Input: part model. Units: mm. Frame: model coordinates. Face numbers are marked on the shaded views. A direction names the side the tool comes from. Round coordinates to 2 decimals unless told otherwise and drop trailing zeros. Loops run counter-clockwise (first coordinate to the right, second up) from the corner with the lowest first, then second, coordinate; pieces in that order, holes last. Notation, with made-up numbers: (-25.75, 84.25) - (-15.75, 84.25) arc R13 ccw to (-15.75, 104.25) - close; hole circle Ø4 at (68, 45.5). An arc over 180 degrees is marked (long way). Write each question's results on one line, items separated by ' | '.
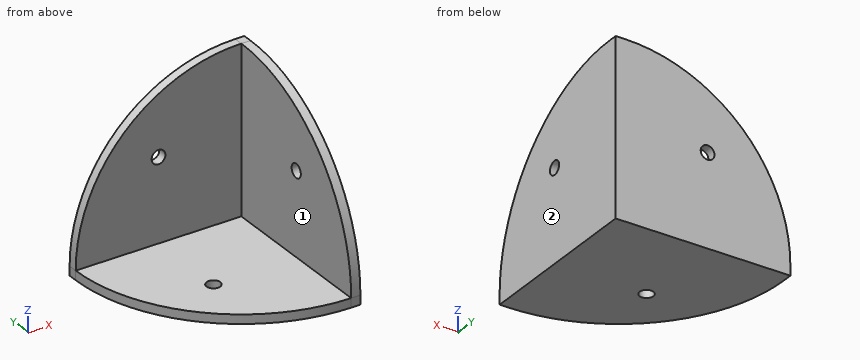
Autodesk Fusion 360 part; units mm, degrees
sketch "Sketch3" plane through (0, 0, 0) normal (0, 0, 1) x (1, 0, 0)
  line L0 (10, 15) -> (46, 15)
  line L1 (46, 15) -> (46, 51)
  line L2 (46, 51) -> (10, 51)
  line L3 (10, 51) -> (10, 15)
  line L4 (8, 53) -> (8, 13)
  line L5 (8, 13) -> (48, 13)
  line L6 (48, 13) -> (48, 53)
  line L7 (48, 53) -> (8, 53)
  line L8 (10, 51) -> (10, 53)
  line L9 (10, 51) -> (8, 51)
  line L10 (46, 51) -> (46, 53)
  line L11 (46, 51) -> (48, 51)
  line L12 (46, 15) -> (48, 15)
  line L13 (46, 15) -> (46, 13)
  line L14 (10, 15) -> (10, 13)
  line L15 (10, 15) -> (8, 15)
  dimension "d6" = 36
  dimension "d7" = 36
  dimension "d8" = 2
extrude "Extrude1" add sketch "Sketch3" along normal blind 38 contours L1 L6 L11 L12 | L2 L7 L8 L10 | L6 L7 L10 L11
extrude "Extrude2" add sketch "Sketch3" along normal blind 2 contours L0 L1 L2 L3
sketch "Sketch4" plane through (0, 0, 2) normal (0, 0, 1) x (-1, 0, 0)
  line L0 (-10, -51) -> (-10, -15)
  line L1 (-10, -15) -> (-46, -15)
  line L2 (-46, -15) -> (-46, -51)
  line L3 (-46, -51) -> (-10, -51)
  line L4 (-10, -51) -> (-46, -15)
  line L5 (-10, -15) -> (-46, -51)
  circle A0 centre (-28, -33) radius 1.5
  dimension "d13" = 3
sketch "Sketch5" plane through (0, 51, 0) normal (0, -1, 0) x (1, 0, 0)
  line L0 (10, 2) -> (46, 2)
  line L1 (46, 2) -> (46, 38)
  line L2 (46, 38) -> (10, 38)
  line L3 (10, 38) -> (10, 2)
  line L4 (10, 38) -> (46, 2)
  line L5 (10, 2) -> (46, 38)
  circle A0 centre (28, 20) radius 1.5
  dimension "d14" = 3
sketch "Sketch6" plane through (46, 0, 0) normal (-1, 0, 0) x (0, -1, 0)
  line L0 (-51, 2) -> (-15, 2)
  line L1 (-15, 2) -> (-15, 38)
  line L2 (-15, 38) -> (-51, 38)
  line L3 (-51, 38) -> (-51, 2)
  line L4 (-51, 38) -> (-15, 2)
  line L5 (-51, 2) -> (-15, 38)
  circle A0 centre (-33, 20) radius 1.5
  dimension "d15" = 3
extrude "Extrude3" cut sketch "Sketch5" against normal blind 7 contours L4 L5 A0 | L4 L5 A0 | L4 L5 A0 | L4 L5 A0
extrude "Extrude4" cut sketch "Sketch6" against normal blind 10 contours L4 L5 A0 | L4 L5 A0 | L4 L5 A0 | L4 L5 A0
extrude "Extrude5" cut sketch "Sketch4" against normal blind 9 contours L4 L5 A0 | L4 L5 A0 | L4 L5 A0 | L4 L5 A0
fillet "Fillet1" radius 36 3 edges at (10, 52, 38) (10, 15, 1) (47, 15, 38)
1. Line query: line 1 (Z direction, x = 18.5, y = 33.5); line 2 (Y direction, x = 28, z = 0.9); line 3 (Y direction, x = 44.5, z = 24). Output: solid intervals per line, ascending. Write a range as [from, to].
Answer:
line 1: [0, 2] | line 2: [19.82, 31.5], [34.5, 53] | line 3: [51, 53]
2. Section query A-A, the plane x = 28. Output: boundary loops of the cut face in (y, z).
Answer:
outline: (19.82, 0) - (31.5, 0) - (31.5, 2) - (19.82, 2) - close; (34.5, 0) - (53, 0) - (53, 18.5) - (51, 18.5) - (51, 2) - (34.5, 2) - close; (51, 21.5) - (53, 21.5) - (53, 33.18) - (51, 33.18) - close
3. Set-up query: the marked faces 1 and 2. Return all of +Z, -Z, +X, -X, +Y, -Y with unobstructed straight access to the full face (end or side cutting, diameter ignored); none if empty.
Answer:
face 1: +Z, -X, -Y | face 2: +Z, -Z, +X, +Y, -Y
4. Section query D-D, the plane x = 15. Output: boundary loops of the cut face in (y, z), plus the area to 3 significant figures.
Answer:
outline: (32.7, 0) - (53, 0) - (53, 20.3) - (51, 20.3) - (51, 2) - (32.7, 2) - close | area: 77.2 mm^2
5. Section query B-B, the plane y = 33. Output: boundary loops of the cut face in (x, z), plus the area to 3 significant figures.
Answer:
outline: (14.82, 0) - (26.5, 0) - (26.5, 2) - (14.82, 2) - close; (29.5, 0) - (48, 0) - (48, 18.5) - (46, 18.5) - (46, 2) - (29.5, 2) - close; (46, 21.5) - (48, 21.5) - (48, 33.18) - (46, 33.18) - close | area: 117 mm^2
6. Section query C-C, the plane y = 29. Output: boundary loops of the cut face in (x, z), plus the area to 3 significant figures.
Answer:
outline: (17.5, 0) - (48, 0) - (48, 30.5) - (46, 30.5) - (46, 2) - (17.5, 2) - close | area: 118 mm^2
7. Contact query for flat-ended pins moving along their axis: pin 1 (1.8 mm diameter, centred on y = 33, z = 20, fed in from -X); pin 2 (5 mm diameter, centred on y = 33.5, z = 12, fed in from -X); pin 3 (2 mm diameter, centred on x = 28.5, z = 12, fed in from -Y); pin 4 (3 mm diameter, centred on x = 16, y = 38, fed in from +Z). Output: stop coordinate, or through.
Answer:
pin 1: through | pin 2: x = 46 | pin 3: y = 51 | pin 4: z = 2
